Model file for the job. Use its own axes, mm. A direction names the side the tool comes from. Round coordinates to 2 decimals unless told otherwise and drop trailing zeros. Order: outer loops, then holes, each group sorted by start corner. A loop starts at its lowest first (then second) coordinate and runs counter-clockwise, first axis right, second up. Notation, with made-up numbers: (-38, 14.25) - (2, 14.25) arc R21 cw to (2, 33.25) - close; hole circle Ø6 at (56, 41.25). An arc over 180 degrees is marked (long way). Use one line per item in the form item = value.
from build123d import *

# Parameters (mm, degrees)
F0_W    = 300
F0_H    = 40
F3_F1_R = 10
F3_F2_R = 10


with BuildPart() as f2:
    # F2: sweep along a path in F1
    with BuildLine(Plane.YZ) as f2_path:
        Line((0, 0), (250, 0))
        Line((250, 0), (250, 200))
    # F0 (on Front) → F2 (sweep)
    with BuildSketch(Plane.XZ):
        with Locations((4.6769320033, 0)):
            Rectangle(F0_W, F0_H)
    sweep(path=f2_path.line, transition=Transition.RIGHT)

    # F3: fillet of radius 10 on 8 edges, made by hand

    # F3_f1
    f3_f1_edges = [f2.edges().sort_by_distance(p)[0] for p in [
        (4.6769320033, 230, 20),
    ]]
    fillet(f3_f1_edges, radius=F3_F1_R)

    # F3_f2
    f3_f2_edges = [f2.edges().sort_by_distance(p)[0] for p in [
        (154.6769320033, 250, 200),
        (-145.3230679967, 250, 200),
        (154.6769320033, 110, 20),
        (4.6769320033, 0, 20),
        (-145.3230679967, 110, 20),
        (4.6769320033, 270, -20),
        (4.6769320033, 230, 200),
        (-145.3230679967, 227.0710678119, 22.9289321881),
        (154.6769320033, 227.0710678119, 22.9289321881),
    ]]
    fillet(f3_f2_edges, radius=F3_F2_R)


solid = f2.part
(1) Tool access for faces 1 (the face through (154.677, 186, 7)), 2 (the face through (7, 255, 200)), 3 (the face through (-142.471, 233.007, 111.12)), 4 (the face through (151.67, 232.85, 111.12)), 5 (the face through (7, 230, 111)): list every direction of +Z, -Z, +X, -X, +Y, -Y with a clear straight run to the whole face (end or side of a thin tool).
Report:
face_1 = +Z, -Z, +X, +Y, -Y
face_2 = +Z, +X, -X, +Y, -Y
face_3 = +Z, -X, -Y
face_4 = +Z, +X, -Y
face_5 = +Z, +X, -X, -Y
(2) Slice it at C-C on z = 151. Give the cut face in (x, y), then the cut area to 3 significant figures.
Report:
outline = (-145.32, 240) arc R10 ccw to (-135.32, 230) - (144.68, 230) arc R10 ccw to (154.68, 240) - (154.68, 270) - (-145.32, 270) - close
area = 12,000 mm2
(3) Probe probe 1 along Z at (x, y) = (-58.5, 41); probe 2 along Y at (x, z) = (-133, 166.5); probe 3 along Z at (x, y) = (-131.5, 232.5). List the from-to ranges inside material, lowest first. Write a range as [from, to].
Report:
probe_1 = [-20, 20]
probe_2 = [230, 270]
probe_3 = [-20, 196.61]
(4) Pin check, flat tips, straight feed: pin 1 (12 mm diameter, centred on x = 21.5, z = 20.5, fed in from -Y); pin 2 (5 mm diameter, centred on x = 117, y = 55, fed in from +Z). Stop position of each tip, or through.
Report:
pin_1 = 1.07
pin_2 = 20
(5) Slice it at B-B on y = 180. Give the cut face in (x, z).
Report:
outline = (-145.32, -20) - (154.68, -20) - (154.68, 10) arc R10 ccw to (144.68, 20) - (-135.32, 20) arc R10 ccw to (-145.32, 10) - close
(6) Slice it at A-A on x = -15. Give the cut face in (y, z).
Report:
outline = (0, -20) - (260, -20) arc R10 ccw to (270, -10) - (270, 200) - (240, 200) arc R10 ccw to (230, 190) - (230, 30) arc R10 cw to (220, 20) - (10, 20) arc R10 ccw to (0, 10) - close
